CAD build for the part. Positions are in the model's coordinates, mm. A direction names the side the tool comes from. Round coordinates to 2 decimals unless told otherwise and drop trailing zeros. Loops run counter-clockwise (first coordinate to the right, second up) from the corner with the lowest first, then second, coordinate; pieces in that order, holes last.
from build123d import *

# Parameters (mm, degrees)
SKETCH1_W        = 515.9375
SKETCH1_H        = 508
SKETCH1_W_2      = 465.1375
SKETCH1_H_2      = 457.2
EXTRUSION1_DEPTH = 2.65684
SKETCH2_W        = 515.9375
SKETCH2_H        = 508
SKETCH2_W_2      = 506.766296236
SKETCH2_H_2      = 498.828796236
EXTRUSION2_DEPTH = 25.4
FILLET1_R        = 3.175


with BuildPart() as part:
    # Sketch1 → Extrusion1 (new body)
    with BuildSketch(Plane.XY):
        Rectangle(SKETCH1_W, SKETCH1_H)
        Rectangle(SKETCH1_W_2, SKETCH1_H_2, mode=Mode.SUBTRACT)
    extrude(amount=EXTRUSION1_DEPTH)

    # Sketch2 → Extrusion2 (add)
    with BuildSketch(Plane.XY.offset(2.65684)):
        Rectangle(SKETCH2_W, SKETCH2_H)
        Rectangle(SKETCH2_W_2, SKETCH2_H_2, mode=Mode.SUBTRACT)
    extrude(amount=EXTRUSION2_DEPTH)

    # Fillet1
    fillet1_edges = [part.edges().sort_by_distance(p)[0] for p in [
        (-253.383148118, -249.414398118, 15.35684),
        (-253.383148118, 249.414398118, 15.35684),
        (253.383148118, 249.414398118, 15.35684),
        (253.383148118, -249.414398118, 15.35684),
        (-253.383148118, 0, 2.65684),
        (0, -249.414398118, 2.65684),
        (253.383148118, 0, 2.65684),
        (0, 249.414398118, 2.65684),
    ]]
    fillet(fillet1_edges, radius=FILLET1_R)


solid = part.part
Item 1: Cut at C-C (z = 17.5). List the corners of the cut face in (x, y) (3 decimals), plus the area to 3 significant figures.
Verdict:
outline: (-257.969, -254) - (257.969, -254) - (257.969, 254) - (-257.969, 254) - close; hole (-253.383, -246.239) arc R3.175 ccw to (-250.208, -249.414) - (250.208, -249.414) arc R3.175 ccw to (253.383, -246.239) - (253.383, 246.239) arc R3.175 ccw to (250.208, 249.414) - (-250.208, 249.414) arc R3.175 ccw to (-253.383, 246.239) - close
area: 9,320 mm2
Item 2: Cut at A-A (y = -179.5). List the corners of the cut face in (x, z) (3 decimals), plus the area to 3 significant figures.
Verdict:
outline: (-257.969, 0) - (-232.569, 0) - (-232.569, 2.657) - (-250.208, 2.657) arc R3.175 cw to (-253.383, 5.832) - (-253.383, 28.057) - (-257.969, 28.057) - close; (232.569, 0) - (257.969, 0) - (257.969, 28.057) - (253.383, 28.057) - (253.383, 5.832) arc R3.175 cw to (250.208, 2.657) - (232.569, 2.657) - close
area: 372 mm2
Item 3: Wall check: L1, parallel to X at y = 80, z = 18.25; L2, parallel to Y at x = 227.5, z = 6.75; L3, parallel to Y at x = -141, z = 2.5. Give the ranges that are in metal, low to high.
Verdict:
L1: x = -257.97 to -253.38, 253.38 to 257.97
L2: y = -254 to -249.41, 249.41 to 254
L3: y = -254 to -228.6, 228.6 to 254
Item 4: Cut at B-B (x = -65). List the corners of the cut face in (y, z) (3 decimals).
Verdict:
outline: (-254, 0) - (-228.6, 0) - (-228.6, 2.657) - (-246.239, 2.657) arc R3.175 cw to (-249.414, 5.832) - (-249.414, 28.057) - (-254, 28.057) - close; (228.6, 0) - (254, 0) - (254, 28.057) - (249.414, 28.057) - (249.414, 5.832) arc R3.175 cw to (246.239, 2.657) - (228.6, 2.657) - close
Item 5: 3-axis set-ups, long thin cutter, end or side, ignore diameter. For faces 4 (the flat face through (-257.969, -4, 14)), 5 (the flat face through (-4, 249.414, 17)): which of +Z, -Z, +X, -X, +Y, -Y reach the whole face in a straight line?
Verdict:
face 4: +Z, -Z, -X, +Y, -Y
face 5: +Z
Item 6: Mould opens along Y. For faces 1 (the flat face through (-4, -254, 14)), 2 (the flat face through (-20, -243, 0)), 3 (the flat face through (253.383, -3, 17)) say: released by +Y, released by -Y, zero draft, split by the parting line, or undercut.
Verdict:
face 1: released by -Y
face 2: zero draft
face 3: undercut
